Geometry: see drawing. Coordinates: mm, zero at the bounding-box minimum. A direction names the side the tool comes from. Give positions to 0.01 mm unless a question says otherwise; leave off trailing zeros. Loops run counter-clockwise (first coordinate to the right, second up) from the corner with the lowest first, then second, coordinate; pieces in that order, holes last. Notation, with made-up numbers: (85, 2) - (121, 2) arc R21 cw to (121, 13) - close; hole circle Ø8 at (75, -8.5). An arc over 180 degrees is marked (long way). One line per question, with ' | ' between items. Start each with the question number.
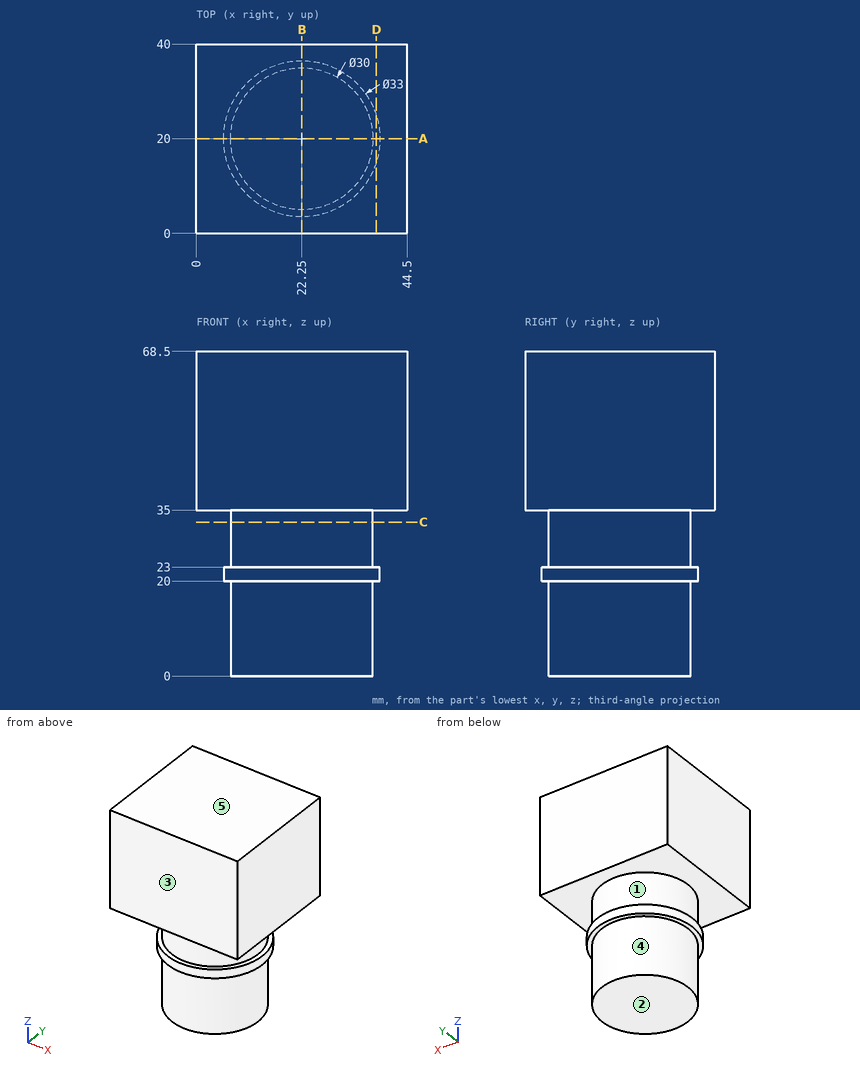
Q1. Line query: L1, parallel to Z at x = 36, y = 26.5; L2, parallel to Z at x = 42.5, y = 5; L3, parallel to X at y = 13.5, z = 14.5. Output: solid intervals per line, ascending. Write a range as from..to.
Q2. Section B-B, the plane x = 22.25. Output: boundary loops of the cut face in (y, z), plus the area to 3 significant figures.
Q3. Section D-D, the plane x = 38. Output: boundary loops of the cut face in (y, z), plus the area to 3 significant figures.
Q4. Section C-C, the plane z = 32.5. Output: boundary loops of the cut face in (x, y).
Q5. Section A-A, the plane y = 20. Output: boundary loops of the cut face in (x, z).
Q6. Access query for the marked faces 4 and 5. Directions: +Z, -Z, +X, -X, +Y, -Y. A direction counts if a zero-diameter tool reaches every point of the face in a straight line with its end or side. Return the directions, or none.
Q7. Draft query along Z for the marked faces 1, 2 and 3. Return one class per face: +Z half, -Z half, draft (parallel to the pull), parting line (faces both ways), or undercut.
Q8. First-contact query: pin 1 (4 mm diameter, centred on x = 11, z = 20, fed in from +Y); pin 2 (5 mm diameter, centred on x = 27, z = 28.5, fed in from +Y); pin 3 (10 mm diameter, centred on y = 31.5, z = 14.5, fed in from -X). Flat tips, straight axial feed; report the tip coordinate or a pass-through.
Solved:
1) L1: z = 20..23, 35..68.5 | L2: z = 35..68.5 | L3: x = 8.73..35.77
2) outline: (0, 35) - (5, 35) - (5, 23) - (3.5, 23) - (3.5, 20) - (5, 20) - (5, 0) - (35, 0) - (35, 20) - (36.5, 20) - (36.5, 23) - (35, 23) - (35, 35) - (40, 35) - (40, 68.5) - (0, 68.5) - close | area: 2,400 mm²
3) outline: (0, 35) - (40, 35) - (40, 68.5) - (0, 68.5) - close; (15.08, 20) - (24.92, 20) - (24.92, 23) - (15.08, 23) - close | area: 1,370 mm²
4) outline: circle Ø30 at (22.25, 20)
5) outline: (0, 35) - (7.25, 35) - (7.25, 23) - (5.75, 23) - (5.75, 20) - (7.25, 20) - (7.25, 0) - (37.25, 0) - (37.25, 20) - (38.75, 20) - (38.75, 23) - (37.25, 23) - (37.25, 35) - (44.5, 35) - (44.5, 68.5) - (0, 68.5) - close
6) face 4: -Z | face 5: +Z, +X, -X, +Y, -Y
7) face 1: undercut | face 2: -Z half | face 3: draft
8) pin 1: stops at y = 33.66 | pin 2: stops at y = 34.83 | pin 3: stops at x = 8.73
